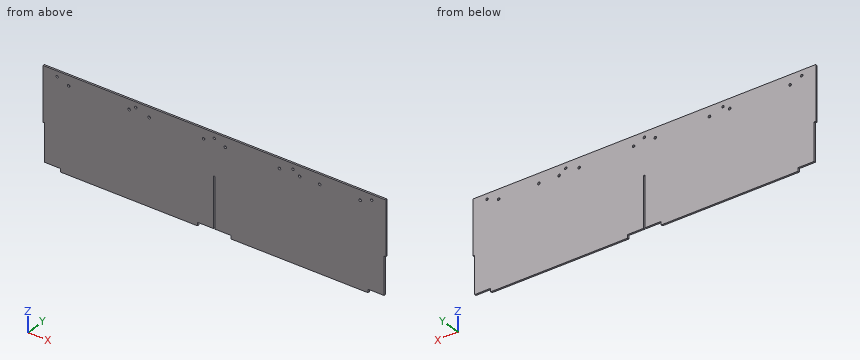
from build123d import *

# Parameters (mm, degrees)
SKETCH1_W            = 629.90984
SKETCH1_H            = 147.69846
BOSS_EXTRUDE1_DEPTH  = 3.175
SKETCH3_W            = 254
SKETCH3_H            = 3.175
BOSS_EXTRUDE2_DEPTH  = 6.35
SKETCH4_W            = 3.175
SKETCH4_H            = 188.732840052
CUT_EXTRUDE1_DEPTH   = 3.175
SKETCH9_W            = 3.175
SKETCH9_H            = 77.20584
BOSS_EXTRUDE4_DEPTH  = 3.175
SKETCH10_W           = 636.25984
SKETCH10_H           = 24.39416
BOSS_EXTRUDE5_DEPTH  = 3.175
SKETCH13_R           = 2.25
CUT_EXTRUDE3_DEPTH   = 652.56536379
M4_CLEARANCE_HOLE1_D = 4.8


with BuildPart() as part:
    # Sketch1 → Boss-Extrude1 (new body)
    with BuildSketch(Plane(origin=(0, 0, 0), x_dir=(1, 0, 0), z_dir=(0, 1, 0))):
        with Locations((314.95492, 73.84923)):
            Rectangle(SKETCH1_W, SKETCH1_H)
    extrude(amount=BOSS_EXTRUDE1_DEPTH)

    # Sketch3 → Boss-Extrude2 (add)
    with BuildSketch(Plane(origin=(0, 0, -147.69846), x_dir=(-1, 0, 0), z_dir=(0, 0, -1))):
        with Locations((-473.22613, 1.5875)):
            Rectangle(SKETCH3_W, SKETCH3_H)
        with Locations((-156.68371, 1.5875)):
            Rectangle(SKETCH3_W, SKETCH3_H)
    extrude(amount=BOSS_EXTRUDE2_DEPTH)

    # Sketch4 → Cut-Extrude1 (cut)
    with BuildSketch(Plane(origin=(0, 3.175, 0), x_dir=(1, 0, 0), z_dir=(0, 1, 0))):
        with Locations((314.95492, 147.69846)):
            Rectangle(SKETCH4_W, SKETCH4_H)
    extrude(amount=-CUT_EXTRUDE1_DEPTH, mode=Mode.SUBTRACT)

    # Sketch9 → Boss-Extrude4 (add, through all)
    with BuildSketch(Plane.XZ):
        with Locations((-1.5875, -38.60292)):
            Rectangle(SKETCH9_W, SKETCH9_H)
        with Locations((631.49734, -38.60292)):
            Rectangle(SKETCH9_W, SKETCH9_H)
    extrude(amount=-BOSS_EXTRUDE4_DEPTH)

    # Sketch10 → Boss-Extrude5 (add, through all)
    with BuildSketch(Plane(origin=(0, 3.175, 0), x_dir=(1, 0, 0), z_dir=(0, 1, 0))):
        with Locations((314.95492, -12.19708)):
            Rectangle(SKETCH10_W, SKETCH10_H)
    extrude(amount=-BOSS_EXTRUDE5_DEPTH)

    # Sketch13 → Cut-Extrude3 (cut, through all)
    with BuildSketch(Plane(origin=(0, 3.175, 0), x_dir=(1, 0, 0), z_dir=(0, 1, 0))):
        with Locations(Location((606.977733219, -14.23416, 0), (0, 0, 270))):
            Circle(SKETCH13_R)
        with Locations(Location((460.966326609, -14.23416, 0), (0, 0, 270))):
            Circle(SKETCH13_R)
        with Locations(Location((314.95492, -14.23416, 0), (0, 0, 270))):
            Circle(SKETCH13_R)
        with Locations(Location((168.943513391, -14.23416, 0), (0, 0, 270))):
            Circle(SKETCH13_R)
        with Locations(Location((22.932106781, -14.23416, 0), (0, 0, 270))):
            Circle(SKETCH13_R)
    extrude(amount=-CUT_EXTRUDE3_DEPTH, mode=Mode.SUBTRACT)

    # M4 Clearance Hole1 (through all)
    with Locations(Plane(origin=(0, 3.175, 0), x_dir=(1, 0, 0), z_dir=(0, 1, 0))):
        with Locations((44.409412743, -5.996840051), (156.68371, -5.996840051), (194.108475752, -5.996840051), (294.859886505, -5.996840051), (335.049953495, -5.996840051), (435.801364248, -5.996840051), (473.22613, -5.996840051), (510.650895752, -5.996840051), (585.500427257, -5.996840051)):
            Hole(M4_CLEARANCE_HOLE1_D / 2)


solid = part.part
Read the model definition and answer for the solid it produces. Units are mm, in the model's axes. Coordinates: 2 decimals unless noted, no trailing zeros. Order: outer loops, then holes, each group sorted by start corner. A loop starts at its lowest first (then second) coordinate and runs counter-clockwise, first axis right, second up. Notation, with made-up numbers: M 11,76.5 L 67,76.5 A11 cw 67,87.5 Z; hole C 30,40 d6. An arc over 180 degrees is marked long. Put each result on its own line as item: value. Start each with the question number.
Item 1: Given pin 1 Ø4 at (x, z) = (179, -64) entering from -Y; pin 2 Ø1.6 at (x, y) = (11.5, 2) entering from -Z; pin 3 Ø1 at (y, z) = (2, -151.5) entering from +X; pin 4 Ø1 at (y, z) = (1.5, -151) entering from -X, each flat-ended and moving along its own axis, determine where each tip first touches the part or whether it passes through.
Item 2: Consider probe 1 along X at (y, z) = (1.6, -136.5); probe 2 along X at (y, z) = (2.4, -54) (3 decimals); probe 3 along Z at (x, y) = (194.5, 0.9). Determine where each line is inside the solid, lowest interval first. Write a range as [from, to].
Item 3: Section B-B, the plane x = 304 is taken. Determine the outline of the cut face in (y, z) (3 decimals), plus the area to 3 significant figures.
Item 4: Section A-A, the plane y = 2.4 is taken. Count the separate pieces of the cut face and the enclosed holes in it, plus the area to 3 significant figures.
Computed:
1. pin 1: stops at y = 0
1. pin 2: stops at z = -147.7
1. pin 3: stops at x = 600.23
1. pin 4: stops at x = 29.68
2. probe 1: x = [0, 313.37], [316.54, 629.91]
2. probe 2: x = [-3.175, 313.367], [316.542, 633.085]
2. probe 3: z = [-154.05, 3.63], [8.36, 24.39]
3. outline: M 0,-147.698 L 3.175,-147.698 L 3.175,24.394 L 0,24.394 Z
3. area: 546 mm2
4. separate pieces: 1
4. enclosed holes: 14
4. area: 112,000 mm2
